Work out the finished part from the listing and answer in its coordinate system (mm). Face numbers are marked on the shaded views. A direction names the side the tool comes from. Round coordinates to 2 decimals unless told otherwise and drop trailing zeros. Order: outer loops, then holes, each group sorted by start corner. A loop starts at its lowest first (then second) coordinate and runs counter-clockwise, first axis right, second up. Notation, with made-up numbers: (65, 1) -> (112, 1) arc R15 cw to (112, 11) -> close; hole circle Ø1 at (54, -30.5). An arc over 180 degrees is marked (long way). Use a Markdown table: item, result. Add a question column.
Item 1: Flat-ended cylindrical pins translate along their axes: P1, Ø3, axis at x = 0, z = 3, coming from the -Y side; P2, Ø3.5, axis at x = 0, z = 3, coming from the +Y side. Find the tip coordinate at first contact, or state that the pin passes through.
Item 2: A cutting plane is placed at C-C, the plane y = -0.35. Determine the outline of the cut face in (x, z), plus the area to 3 significant figures.
Item 3: A cutting plane is placed at D-D, the plane y = -2.35. Determine the outline of the cut face in (x, z), plus the area to 3 significant figures.
Item 4: For a pull along X with two mould halves and no side action, classify the marked faces 1, 2, 3 and 4 as +X half, -X half, draft (parallel to the pull), parting line (faces both ways), or undercut.
Item 5: A tool of negligible diameter and unlimited length cuts with its end or side. For the marked faces 5 and 6, from which of +Z, -Z, +X, -X, +Y, -Y can it reach the whole face along a straight path? Write none if from no direction.
Item 6: A cutting plane is placed at B-B, the plane x = 0. Determine the outline of the cut face in (y, z), plus the area to 3 significant figures.
Item 7: A cutting plane is placed at A-A, the plane z = 3. Determine the outline of the cut face in (x, y), plus the area to 3 significant figures.
Item 8: Find the intervals of material crossed by L1, parallel to Z at x = 0, y = -1.05; L2, parallel to X at y = -3, z = 3.25; L3, parallel to Z at x = -1.75, y = -3.2, in increasing order. Write a range as [from, to].
from build123d import *

# Parameters (mm, degrees)
PAD_DEPTH       = 6
SKETCH001_R     = 1.6
POCKET_DEPTH    = 4.001
POCKET001_DEPTH = 2.36
FILLET_R        = 0.1


with BuildPart() as part:
    # Sketch → Pad (new body)
    with BuildSketch(Plane.XY):
        Polygon((0, 0), (-5.44, 0), (-5.44, -1.68), (-2.94, -4), (0, -4), (2.94, -4), (5.44, -1.68), (5.44, 0), align=None)
    extrude(amount=PAD_DEPTH)

    # Sketch001 (on Face5 of Pad) → Pocket (cut, through all)
    with BuildSketch(Plane.XZ.offset(4)):
        with Locations((0, 3)):
            Circle(SKETCH001_R)
    extrude(amount=-POCKET_DEPTH, mode=Mode.SUBTRACT)

    # Sketch002 (on Face8 of Pocket) → Pocket001 (cut)
    with BuildSketch(Plane.XZ.offset(4)):
        Polygon((-2.87, 4.656995), (-2.87, 1.343005), (0, -0.313991), (2.87, 1.343005), (2.87, 4.656995), (0, 6.313991), align=None)
    extrude(amount=-POCKET001_DEPTH, mode=Mode.SUBTRACT)

    # Fillet
    fillet_edges = [part.edges().sort_by_distance(p)[0] for p in [
        (-0.543848, -2.82, 6),
        (0.543848, -2.82, 6),
        (0.543848, -2.82, 0),
        (-0.543848, -2.82, 0),
    ]]
    fillet(fillet_edges, radius=FILLET_R)


solid = part.part
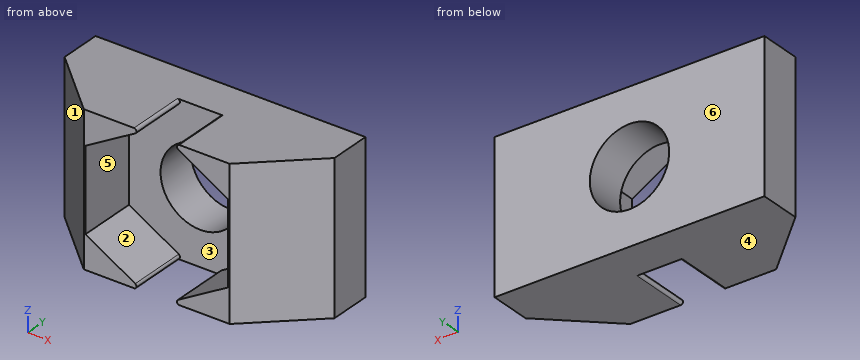
Reported:
| question | item | result |
|---|---|---|
| 1 | P1 | through |
| 1 | P2 | y = 0 |
| 2 | outline | (-5.44, 0) -> (5.44, 0) -> (5.44, 6) -> (-5.44, 6) -> close; hole circle Ø3.2 at (0, 3) |
| 2 | area | 57.2 mm² |
| 3 | outline | (-4.72, 0) -> (-0.92, 0) arc R0.1 ccw to (-0.87, 0.19) -> (-2.87, 1.34) -> (-2.87, 4.66) -> (-0.87, 5.81) arc R0.1 ccw to (-0.92, 6) -> (-4.72, 6) -> close; (0.87, 0.19) arc R0.1 ccw to (0.92, 0) -> (4.72, 0) -> (4.72, 6) -> (0.92, 6) arc R0.1 ccw to (0.87, 5.81) -> (2.87, 4.66) -> (2.87, 1.34) -> close |
| 3 | area | 28.3 mm² |
| 4 | face 1 | -X half |
| 4 | face 2 | undercut |
| 4 | face 3 | undercut |
| 4 | face 4 | draft |
| 5 | face 5 | -Y |
| 5 | face 6 | +Z, -Z, +X, -X, +Y |
| 6 | outline | (-1.64, 0) -> (0, 0) -> (0, 1.4) -> (-1.64, 1.4) -> close; (-1.64, 4.6) -> (0, 4.6) -> (0, 6) -> (-1.64, 6) -> close |
| 6 | area | 4.59 mm² |
| 7 | outline | (-5.44, -1.68) -> (-2.94, -4) -> (-2.87, -4) -> (-2.87, -1.64) -> (-1.6, -1.64) -> (-1.6, 0) -> (-5.44, 0) -> close; (1.6, -1.64) -> (2.87, -1.64) -> (2.87, -4) -> (2.94, -4) -> (5.44, -1.68) -> (5.44, 0) -> (1.6, 0) -> close |
| 7 | area | 18.9 mm² |
| 8 | L1 | [0, 1.4], [4.6, 6] |
| 8 | L2 | [-4.02, -2.87], [2.87, 4.02] |
| 8 | L3 | [0, 0.7], [5.3, 6] |
